Geometry: final body of the model. Coordinates: model frame, mm. A direction names the side the tool comes from. Give positions to 0.01 mm unless a question says otherwise; leave off trailing zeros. Loops run counter-clockwise (first coordinate to the right, second up) from the corner with the lowest first, then second, coordinate; pieces in that order, holes last. Notation, with made-up numbers: (12.25, -35.75) -> (38.25, -35.75) arc R17 cw to (38.25, -29.75) -> close; hole circle Ø3 at (7, 87). An arc over 180 degrees is marked (long way). One line per item, written item: value. Start each with the question number.
Autodesk Inventor part; units mm, degrees
ref_plane "YZ Plane" through (0, 0, 0) normal (1, 0, 0) x (0, 1, 0)
ref_plane "XZ Plane" through (0, 0, 0) normal (0, 1, 0) x (-1, 0, 0)
ref_plane "XY Plane" through (0, 0, 0) normal (0, 0, 1) x (1, 0, 0)
sketch "Sketch1" plane through (0, 0, 0) normal (0, 1, 0) x (-1, 0, 0)
  line L0 (349.8743, 0) -> (258.4057, -158.4282)
  line L1 (174.9371, -303) -> (-174.9371, -303)
  line L2 (-174.9371, -303) -> (-349.8743, 0)
  line L3 (-349.8743, 0) -> (-174.9371, 303)
  line L4 (-174.9371, 303) -> (174.9371, 303)
  line L5 (258.4057, 158.4282) -> (349.8743, 0)
  line L6 (0, 0) -> (-8, 0)
  line L7 (-8, 0) -> (-8, -303)
  line L8 (-8, -303) -> (8, -303)
  line L9 (8, -303) -> (8, 0)
  line L10 (8, 0) -> (-8, 0)
  circle A0 centre (0, 0) radius 2.5
  line L11 (258.4057, 158.4282) -> (-4, 6.9282)
  line L12 (4, -6.9282) -> (266.4057, 144.5718)
  line L13 (-4, 6.9282) -> (4, -6.9282)
  line L14 (-266.4057, 144.5718) -> (-4, -6.9282)
  line L15 (4, 6.9282) -> (-258.4057, 158.4282)
  line L16 (-4, -6.9282) -> (4, 6.9282)
  line L17 (8, -4.6188) -> (8, -151.5)
  line L18 (8, -151.5) -> (-8, -151.5)
  line L19 (-8, -151.5) -> (-8, -303)
  line L20 (-8, -4.6188) -> (-4, -6.9282)
  line L21 (4, -6.9282) -> (-4, -6.9282)
  line L22 (-266.4057, 144.5718) -> (-258.4057, 158.4282)
  line L23 (-127.2028, 82.6782) -> (-135.2028, 68.8218)
  line L24 (-135.2028, 68.8218) -> (-8, -4.6188)
  line L25 (-266.4057, 144.5718) -> (-349.8743, 0)
  line L26 (-174.9371, -303) -> (-349.8743, 0)
  line L27 (-174.9371, -303) -> (-8, -303)
  line L28 (0, 9.2376) -> (8, 0)
  dimension "d0" = 303
  dimension "d1" = 303
  dimension "d2" = 8
  dimension "d3" = 16
  dimension "d4" = 5
  dimension "d7" = 360
extrude "Extrusion1" add sketch "Sketch1" along normal blind 3 contours L1 L7 L18 L9 | L1 L2 L3 L14 L7 | L18 L7 L14 L21 L12 L9 | L12 L13 A0 L10 L9 | L14 L23 L15 L11 L13 A0 L6 L7 | L7 L6 A0 L16 L14 | L10 A0 L16 L28 | L21 L16 A0 L13 | L3 L15 L23 L14 | A0 L13 L10 | L10 L16 A0 | L28 L15 L16 | L16 A0 L13 L11 L28 | A0 L16 L13 | A0 L13 L6 | L6 L16 A0 | L13 A0 L16
sketch "Sketch2" plane through (0, 3, 0) normal (0, 1, 0) x (1, 0, 0)
  line L0 (-8, 303) -> (-8, 0)
  line L1 (-8, 0) -> (-8, 151.5)
  line L2 (-8, 151.5) -> (8, 151.5)
  line L3 (8, 151.5) -> (8, 0)
  line L4 (8, 0) -> (-8, 0)
  line L5 (0, -9.2376) -> (258.4057, -158.4282)
  line L6 (258.4057, -158.4282) -> (126.3368, -82.1782)
  line L7 (126.3368, -82.1782) -> (134.8368, -67.4558)
  line L8 (134.8368, -67.4558) -> (266.9057, -143.7058)
  line L9 (266.9057, -143.7058) -> (258.4057, -158.4282)
  point P0 (0, 0)
  dimension "d11" = 151.5
  dimension "d12" = 16
  dimension "d13" = 152.5
  dimension "d14" = 17
extrude "Extrusion2" cut sketch "Sketch2" against normal blind 3
sketch "Sketch3" plane through (0, 3, 0) normal (0, 1, 0) x (1, 0, 0)
  line L0 (174.9371, 303) -> (-8, 303)
  line L1 (174.9371, 303) -> (149.9371, 303)
  line L2 (149.9371, 303) -> (149.9371, 297)
  line L3 (149.9371, 297) -> (174.9371, 297)
  line L4 (174.9371, 297) -> (174.9371, 303)
  line L5 (349.8743, 0) -> (174.9371, 303)
  line L6 (174.9371, 303) -> (187.4371, 281.3494)
  line L7 (187.4371, 281.3494) -> (182.241, 278.3494)
  line L8 (182.241, 278.3494) -> (169.741, 300)
  line L9 (169.741, 300) -> (174.9371, 303)
  line L10 (349.8743, 0) -> (337.3743, 21.6506)
  line L11 (337.3743, 21.6506) -> (332.1781, 18.6506)
  line L12 (332.1781, 18.6506) -> (344.6781, -3)
  line L13 (344.6781, -3) -> (349.8743, 0)
  line L14 (349.8743, 0) -> (337.3743, -21.6506)
  line L15 (337.3743, -21.6506) -> (332.1781, -18.6506)
  line L16 (332.1781, -18.6506) -> (344.6781, 3)
  line L17 (344.6781, 3) -> (349.8743, 0)
  line L18 (349.8743, 0) -> (266.9057, -143.7058)
  line L19 (349.8743, 0) -> (374.8743, 0) construction
  point P0 (0, 0)
  dimension "d17" = 25
  dimension "d18" = 6
  dimension "d19" = 25
  dimension "d20" = 6
  dimension "d21" = 25
  dimension "d22" = 6
  dimension "d23" = 25
  dimension "d24" = 120
  dimension "d25" = 6
extrude "Extrusion3" cut sketch "Sketch3" against normal blind 3
sketch "Sketch4" plane through (0, 3, 0) normal (0, 1, 0) x (1, 0, 0)
  line L0 (-55.0368, 49.6734) -> (70.5368, -22.8266)
  line L1 (70.5368, -22.8266) -> (55.0368, -49.6734)
  line L2 (55.0368, -49.6734) -> (-70.5368, 22.8266)
  line L3 (-70.5368, 22.8266) -> (-55.0368, 49.6734)
  line L4 (-55.0368, 49.6734) -> (55.0368, -49.6734) construction
  line L5 (70.5368, -22.8266) -> (-70.5368, 22.8266) construction
  line L6 (-55.0368, 49.6734) -> (89.9632, 49.6734) construction
  line L7 (-15.5, -72.5) -> (-15.5, 72.5)
  line L8 (-15.5, 72.5) -> (15.5, 72.5)
  line L9 (15.5, 72.5) -> (15.5, -72.5)
  line L10 (15.5, -72.5) -> (-15.5, -72.5)
  line L11 (-15.5, -72.5) -> (15.5, 72.5) construction
  line L12 (-15.5, 72.5) -> (15.5, -72.5) construction
  line L13 (-8, 0) -> (8, 0)
  line L14 (-15.5, -72.5) -> (129.5, -72.5) construction
  point P0 (0, 0)
  dimension "d28" = 145
  dimension "d29" = 30
  dimension "d30" = 31
  dimension "d31" = 145
  dimension "d32" = 90
  dimension "d33" = 31
extrude "Extrusion4" cut sketch "Sketch4" against normal blind 3
sketch "Sketch5" plane through (0, 3, 0) normal (0, 1, 0) x (1, 0, 0)
  line L0 (-1, 151.5) -> (-1, 191.5)
  circle A0 centre (-1, 191.5) radius 2.75
  circle A1 centre (-1, 231.5) radius 2.75
  circle A2 centre (-1, 271.5) radius 2.75
  circle A3 centre (0, 0) radius 0.5
  line L1 (126.3368, -82.1782) -> (134.8368, -67.4558)
  line L2 (126.3368, -82.1782) -> (129.3368, -76.9821)
  line L3 (129.3368, -76.9821) -> (103.3561, -61.9821)
  line L4 (103.3561, -61.9821) -> (77.3753, -46.9821)
  circle A4 centre (103.3561, -61.9821) radius 2.75
  circle A5 centre (77.3753, -46.9821) radius 2.75
  line L5 (-8, 303) -> (-8, 151.5)
  dimension "d36" = 40
  dimension "d37" = 5.5
  dimension "d40" = 40
  dimension "d45" = 1
  dimension "d46" = 6
  dimension "d47" = 30
  dimension "d48" = 30
  dimension "d49" = 5.5
  dimension "d50" = 5.5
  dimension "d53" = 7
extrude "Extrusion5" cut sketch "Sketch5" against normal blind 3 contours A0 | A1 | A2 | A4 L4 L3 | A5 | L3 L4 A4
sketch "Sketch6" plane through (0, 3, 0) normal (0, 1, 0) x (1, 0, 0)
  line L0 (-8, 303) -> (-8, 151.5)
  line L1 (-8, 303) -> (344, 303)
  line L2 (344, 303) -> (344, -147)
  line L3 (344, -147) -> (-8, -147)
  line L4 (-8, -147) -> (-8, 303)
  point P0 (0, 0)
  dimension "d54" = 352
  dimension "d55" = 450
properties part number "Acrylic_bottom"
Item 1: Ray query, line 1 along Z through (x, y) = (-1, 1.7); line 2 along X through (y, z) = (2.35, -271.5); line 3 along X through (y, z) = (2.1, -191.5). Return the intervals inside material, ascending. Write a range as [from, to].
Item 2: Pin query (flat end, axial travel): pin 1 (1.5 mm diameter, centred on y = 1.5, z = -301, fed in from +X); pin 2 (1.5 mm diameter, centred on x = 238, y = 2.5, fed in from +Z); pin 3 (1 mm diameter, centred on x = 29.5, y = 0.5, fed in from +Z). Return the tip coordinate at first contact, or that it passes through.
Item 3: Section B-B, the plane x = 218. Output: boundary loops of the cut face in (y, z).
Item 4: Access query for faces 5 (the face through (42.633, 1.521, 6.716)), 6 (the face through (337.487, 1.521, -9.456)), 7 (the face through (170, 0, -77)), 8 (the face through (261.356, 1.479, -153.318)), 9 (the face through (199.95, 1.52, 105.05)). Directions: +Z, -Z, +X, -X, +Y, -Y. A direction counts if a zero-diameter tool reaches every point of the face in a straight line with its end or side. Return the directions, or none.
Item 5: Section A-A, the plane y = 0.7. Output: boundary loops of the cut face in (x, z).
Item 6: Mould query, pull axis Z, two halves, no side actions, for faces 1 (the face through (64.744, 1.521, 32.86)), 2 (the face through (170, 3, -77)), 3 (the face through (337.487, 1.521, 9.456)), 4 (the face through (92.089, 1.479, 62.405)). Classes: pulls with the +Z half, pulls with the -Z half, needs draft (parallel to the pull), parting line crosses it, or undercut.
Item 7: Section C-C, the plane z = -241. Output: boundary loops of the cut face in (x, y).
Geometry check:
1. line 1: z = [-303, -274.25], [-268.75, -234.25], [-228.75, -194.25], [-188.75, -151.5]
1. line 2: x = [-8, -3.75], [1.75, 193.12]
1. line 3: x = [-8, -3.75], [1.75, 239.31]
2. pin 1: stops at x = 149.94
2. pin 2: stops at z = 127.45
2. pin 3: stops at z = -0.58
3. outline: (0, -228.41) -> (3, -228.41) -> (3, 115.47) -> (0, 115.47) -> close
4. face 5: -X, +Y, -Y
4. face 6: +X, +Y, -Y
4. face 7: +Z, -Z, +X, -X, -Y
4. face 8: -Z, +X, +Y, -Y
4. face 9: +Z, +Y, -Y
5. outline: (-8, -303) -> (149.94, -303) -> (149.94, -297) -> (171.47, -297) -> (182.24, -278.35) -> (187.44, -281.35) -> (337.37, -21.65) -> (332.18, -18.65) -> (342.95, 0) -> (332.18, 18.65) -> (337.37, 21.65) -> (266.91, 143.71) -> (134.84, 67.46) -> (126.34, 82.18) -> (58.79, 43.18) -> (70.54, 22.83) -> (15.5, -8.95) -> (15.5, -72.5) -> (8, -72.5) -> (8, -151.5) -> (-8, -151.5) -> close; hole circle Ø5.5 at (-1, -271.5); hole circle Ø5.5 at (-1, -231.5); hole circle Ø5.5 at (-1, -191.5); hole circle Ø5.5 at (77.38, 46.98); hole circle Ø5.5 at (103.36, 61.98)
6. face 1: undercut
6. face 2: needs draft
6. face 3: undercut
6. face 4: pulls with the +Z half
7. outline: (-8, 0) -> (210.73, 0) -> (210.73, 3) -> (-8, 3) -> close
